Check sheet for the modelled part. Datum: model origin and axes. Units: mm. A direction names the side the tool comes from. Give positions to 0.01 mm unless a question says otherwise; leave off trailing zeros. Write each loop counter-clockwise with the first axis right and the second up, starting at its lowest first coordinate (ties: lowest second). Pieces come first, ordered by that corner, then holes. Notation, with made-up numbers: (76, -21) -> (98, -21) arc R19 cw to (98, 12) -> close; hole circle Ø6 at (41, 57.25). An arc over 180 degrees is marked (long way). Return JSON: item names as keys, results as strings.
from build123d import *

# Parameters (mm, degrees)
F0_W     = 120
F0_H     = 40
F1_DEPTH = 10
F2_W     = 100
F2_H     = 20
F3_DEPTH = 5
F4_R     = 4
F5_W     = 100
F5_H     = 12
F6_DEPTH = 5
F7_R     = 4


with BuildPart() as f1:
    # F0 (on Top) → F1 (new body)
    with BuildSketch(Plane.XY):
        Rectangle(F0_W, F0_H)
    extrude(amount=F1_DEPTH)

    # F2 (on face) → F3 (cut)
    with BuildSketch(Plane.XY.offset(10)):
        Rectangle(F2_W, F2_H)
    extrude(amount=-F3_DEPTH, mode=Mode.SUBTRACT)

    # F4
    f4_edges = [f1.edges().sort_by_distance(p)[0] for p in [
        (-50, 10, 7.5),
        (50, 10, 7.5),
        (50, -10, 7.5),
        (-50, -10, 7.5),
    ]]
    fillet(f4_edges, radius=F4_R)

    # F5 (on face) → F6 (cut, through all)
    with BuildSketch(Plane.XY.offset(5)):
        Rectangle(F5_W, F5_H)
    extrude(amount=-F6_DEPTH, mode=Mode.SUBTRACT)

    # F7
    f7_edges = [f1.edges().sort_by_distance(p)[0] for p in [
        (-50, 6, 2.5),
        (-50, -6, 2.5),
        (50, -6, 2.5),
        (50, 6, 2.5),
    ]]
    fillet(f7_edges, radius=F7_R)


solid = f1.part
(1) Cross-section at B-B on x = -34. Enter the section's corners in (y, z).
Reply:
{"outline": "(-20, 0) -> (-6, 0) -> (-6, 5) -> (-10, 5) -> (-10, 10) -> (-20, 10) -> close; (6, 0) -> (20, 0) -> (20, 10) -> (10, 10) -> (10, 5) -> (6, 5) -> close"}
(2) Release check for a two-part mould opening along X. For faces 4 (the flat face through (-1, 20, 5)), 5 (the flat face through (-60, 0, 5)), 6 (the cylindrical face through (48.859, 8.797, 7.465)) record: pulls with the +X half, pulls with the -X half, needs draft (parallel to the pull), parting line crosses it, or undercut.
Reply:
{"face 4": "needs draft", "face 5": "pulls with the -X half", "face 6": "undercut"}
(3) Cross-section at A-A on z = 3.75. Enter the section's corners in (x, y).
Reply:
{"outline": "(-60, -20) -> (60, -20) -> (60, 20) -> (-60, 20) -> close; hole (-50, -2) arc R4 ccw to (-46, -6) -> (46, -6) arc R4 ccw to (50, -2) -> (50, 2) arc R4 ccw to (46, 6) -> (-46, 6) arc R4 ccw to (-50, 2) -> close"}
(4) Set-up check for faces 1 (the flat face through (50, 0, 6)), 2 (the flat face through (-1, -6, 3)), 3 (the flat face through (-1, 9, 0)): record each of +Z, -Z, +X, -X, +Y, -Y from which the full face is reachable in a straight line by a thin tool's end or side.
Reply:
{"face 1": "+Z", "face 2": "+Z, -Z", "face 3": "-Z, +X, -X, +Y, -Y"}
(5) Depth check by flat-ended pin: pin 1 Ø4 at (x, y) = (10.5, -4.5) entering from +Z; pin 2 Ø1 at (x, y) = (-33, 10) entering from -Z. Enter the tip coordinate at first touch or a pass-through.
Reply:
{"pin 1": "z = 5", "pin 2": "z = 0"}
(6) Thickness scan on L1, parallel to Y at x = 3, z = 4.75; L2, parallel to Y at x = 9, z = 7; L3, parallel to X at y = 3, z = 7.25. Record the ranges inside material, lowest first.
Reply:
{"L1": "-20 to -6, 6 to 20", "L2": "-20 to -10, 10 to 20", "L3": "-60 to -50, 50 to 60"}
